```python
from build123d import *

# Parameters (mm, degrees)
F0_R     = 12.7
F0_R_2   = 3.255
F1_DEPTH = 25
F2_R     = 4.900418
F3_DEPTH = 3.25
F4_R     = 0.1
F5_SIZE  = 0.1


with BuildPart() as f1:
    # F0 (on Top) → F1 (new body)
    with BuildSketch(Plane.XY):
        Circle(F0_R)
        Circle(F0_R_2, mode=Mode.SUBTRACT)
    extrude(amount=-F1_DEPTH)

    # F2 (on face) → F3 (cut)
    with BuildSketch(Plane.XY):
        Circle(F2_R)
    extrude(amount=-F3_DEPTH, mode=Mode.SUBTRACT)

    # F4
    f4_edges = [f1.edges().sort_by_distance(p)[0] for p in [
        (-4.900418, 0, -3.25),
    ]]
    fillet(f4_edges, radius=F4_R)

    # F5
    f5_edges = [f1.edges().sort_by_distance(p)[0] for p in [
        (-3.255, 0, -3.25),
        (-4.900418, 0, 0),
        (-3.255, 0, -25),
        (-12.7, 0, -25),
    ]]
    chamfer(f5_edges, length=F5_SIZE)


solid = f1.part
```
Verification items for the finished model (mm, model axes). A direction names the side the tool comes from. Round coordinates to 2 decimals unless told otherwise and drop trailing zeros. Write each loop counter-clockwise with the first axis right and the second up, starting at its lowest first coordinate (ties: lowest second). Pieces come first, ordered by that corner, then holes.
1. Access from +Z, -Z, +X, -X, +Y, -Y to the whole of each face (thin tool, end or side, straight path). Record for faces 4 (the flat face through (2, -3, -3.25)), 5 (the flat face through (5.5, 0.2, 0)).
2. Scan lines: L1, parallel to Y at x = 0, z = -1.8; L2, parallel to Y at x = -0.25, z = -14.5; L3, parallel to X at y = 0.5, z = -11.25. Record each from-to range of solid material in increasing order.
3. Section check A-A on y = 0. Enter the section's corners in (x, z) (3 decimals), plus the area to 3 significant figures.
4. Section check C-C on z = -15. Enter the section's corners in (x, y) (3 decimals).
5. Gauge pin test, flat ends, axial feed: P1, Ø5, axis at x = 0, y = 0, coming from the +Z side; P2, Ø1, axis at x = 4, z = -20, coming from the -Y side; P3, Ø6, axis at x = 9.5, z = -11, coming from the -Y side; P4, Ø10, axis at y = 9, z = -21, coming from the +X side. Record the tip position at first contact, or that the pin passes through.
6. Draft check along X on faces 1 (the flat face through (3, -3, -25)), 2 (the cylindrical face through (-3.89, -2.98, -1.6)), 3 (the cylindrical face through (-2.75, -12.4, -12.28)). Enter one of: +X half, -X half, draft (parallel to the pull), parting line (faces both ways), or undercut.
Answer:
1. face 4: +Z
1. face 5: +Z, +X, -X, +Y, -Y
2. L1: y = -12.7 to -4.9, 4.9 to 12.7
2. L2: y = -12.7 to -3.25, 3.25 to 12.7
2. L3: x = -12.69 to -3.22, 3.22 to 12.69
3. outline: (-12.7, -24.9) - (-12.6, -25) - (-3.355, -25) - (-3.255, -24.9) - (-3.255, -3.35) - (-3.355, -3.25) - (-4.8, -3.25) arc R0.1 cw to (-4.9, -3.15) - (-4.9, -0.1) - (-5, 0) - (-12.7, 0) - close; (3.255, -24.9) - (3.355, -25) - (12.6, -25) - (12.7, -24.9) - (12.7, 0) - (5, 0) - (4.9, -0.1) - (4.9, -3.15) arc R0.1 cw to (4.8, -3.25) - (3.355, -3.25) - (3.255, -3.35) - close
3. area: 462 mm2
4. outline: circle Ø25.4 at (0, 0); hole circle Ø6.51 at (0, 0)
5. P1: passes through
5. P2: stops at y = -12.21
5. P3: stops at y = -10.91
5. P4: stops at x = 12.05
6. face 1: draft
6. face 2: undercut
6. face 3: parting line
